from build123d import *
from build123d.topology import SkipClean

# Parameters (mm, degrees)
SKETCH_2_R             = 3
EXTRUDE_1_DEPTH        = 16.5
EXTRUDE_1_2_DEPTH      = 16.5
EXTRUDE_1_3_DEPTH      = 16.5
EXTRUDE_1_4_DEPTH      = 16.5
SKETCH_3_R             = 1.2
EXTRUDE_2_DEPTH        = 5
SKETCH_4_R             = 5
EXTRUDE_3_DEPTH        = 3
EXTRUDE_3_2_DEPTH      = 3
EXTRUDE_3_3_DEPTH      = 3
EXTRUDE_3_4_DEPTH      = 3
EXTRUDE_4_DEPTH        = 3
EXTRUDE_4_DEPTH_BACK   = 15
SKETCH_6_R             = 5
EXTRUDE_5_DEPTH        = 3
EXTRUDE_5_DEPTH_BACK   = 15
EXTRUDE_5_2_DEPTH      = 3
EXTRUDE_5_2_DEPTH_BACK = 15
EXTRUDE_6_DEPTH        = 3
SKETCH_9_R             = 1.9
EXTRUDE_7_DEPTH        = 4
SKETCH_10_R            = 1.9
EXTRUDE_8_DEPTH        = 4
CHAMFER_1_SIZE         = 1
SKETCH_11_R            = 5
EXTRUDE_9_DEPTH        = 5
SKETCH_12_R            = 2.1
CUT_EXTRUDE_1_DEPTH    = 5
SKETCH_13_R            = 2.1
CUT_EXTRUDE_2_DEPTH    = 4
CHAMFER_2_SIZE         = 1
CHAMFER_3_SIZE         = 0.5


with BuildPart() as part:
    # Sketch 2 → Extrude 1 (new body)
    with BuildSketch(Plane(origin=(0, 0, 0), x_dir=(1, 0, 0), z_dir=(0, 1, 0))):
        with Locations(Location((25, 35, 0), (0, 0, 270))):
            Circle(SKETCH_2_R)
    extrude(amount=EXTRUDE_1_DEPTH)



with BuildPart() as body_2:
    # Sketch 2 → Extrude 1 2 (new body)
    with BuildSketch(Plane(origin=(0, 0, 0), x_dir=(1, 0, 0), z_dir=(0, 1, 0))):
        with Locations(Location((31, -22, 0), (0, 0, 270))):
            Circle(SKETCH_2_R)
    extrude(amount=EXTRUDE_1_2_DEPTH)


with BuildPart() as body_3:
    # Sketch 2 → Extrude 1 3 (new body)
    with BuildSketch(Plane(origin=(0, 0, 0), x_dir=(1, 0, 0), z_dir=(0, 1, 0))):
        with Locations(Location((-31, -22, 0), (0, 0, 90))):
            Circle(SKETCH_2_R)
    extrude(amount=EXTRUDE_1_3_DEPTH)


with BuildPart() as body_4:
    # Sketch 2 → Extrude 1 4 (new body)
    with BuildSketch(Plane(origin=(0, 0, 0), x_dir=(1, 0, 0), z_dir=(0, 1, 0))):
        with Locations(Location((-25, 35, 0), (0, 0, 90))):
            Circle(SKETCH_2_R)
    extrude(amount=EXTRUDE_1_4_DEPTH)


with BuildPart() as part_1:
    add(part.part)

    add(body_2.part)  # Extrude 2 merges body 2

    add(body_3.part)  # Extrude 2 merges body 3

    add(body_4.part)  # Extrude 2 merges body 4
    # Sketch 3 → Extrude 2 (add)
    with BuildSketch(Plane(origin=(0, 16.5, 0), x_dir=(1, 0, 0), z_dir=(0, 1, 0))):
        with Locations(Location((-31, -22, 0), (0, 0, 270))):
            Circle(SKETCH_3_R)
        with Locations(Location((-25, 35, 0), (0, 0, 270))):
            Circle(SKETCH_3_R)
        with Locations(Location((25, 35, 0), (0, 0, 270))):
            Circle(SKETCH_3_R)
        with Locations(Location((31, -22, 0), (0, 0, 270))):
            Circle(SKETCH_3_R)
    extrude(amount=EXTRUDE_2_DEPTH)

    # Sketch 6 → Extrude 4 (add, two sides: drawn at the far end of the back side and taken through both)
    with BuildSketch(Plane(origin=(0, 0, 0), x_dir=(1, 0, 0), z_dir=(0, 1, 0)).offset(-EXTRUDE_4_DEPTH_BACK)):
        with Locations(Location((-28.159807037, -19, 0), (0, 0, 270))):
            Circle(SKETCH_6_R)
        with Locations(Location((28.159807037, -19, 0), (0, 0, 276.602489978))):
            Circle(SKETCH_6_R)
    extrude(amount=EXTRUDE_4_DEPTH + EXTRUDE_4_DEPTH_BACK)



with BuildPart() as body_2_2:
    # Sketch 4 → Extrude 3 (new body)
    with BuildSketch(Plane.XZ):
        with Locations(Location((-25, -15, 0), (0, 0, 270))):
            Circle(SKETCH_4_R)
    extrude(amount=-EXTRUDE_3_DEPTH)


with BuildPart() as body_3_2:
    # Sketch 4 → Extrude 3 2 (new body)
    with BuildSketch(Plane.XZ):
        with Locations(Location((-25, -75, 0), (0, 0, 270))):
            Circle(SKETCH_4_R)
    extrude(amount=-EXTRUDE_3_2_DEPTH)


with BuildPart() as body_4_2:
    # Sketch 4 → Extrude 3 3 (new body)
    with BuildSketch(Plane.XZ):
        with Locations(Location((25, -15, 0), (0, 0, 90))):
            Circle(SKETCH_4_R)
    extrude(amount=-EXTRUDE_3_3_DEPTH)


with BuildPart() as body_5:
    # Sketch 4 → Extrude 3 4 (new body)
    with BuildSketch(Plane.XZ):
        with Locations(Location((33, -75, 0), (0, 0, 270))):
            Circle(SKETCH_4_R)
    extrude(amount=-EXTRUDE_3_4_DEPTH)


with BuildPart() as body_6:
    # Sketch 7 → Extrude 5 (new, two sides: drawn at the far end of the back side and taken through both)
    with BuildSketch(Plane(origin=(0, 0, 0), x_dir=(1, 0, 0), z_dir=(0, 1, 0)).offset(-EXTRUDE_5_DEPTH_BACK)):
        with BuildLine():
            Line((32.175491387, -57.49808516), (25.273954776, -60.367671435))
            ThreePointArc((25.273954776, -60.367671435), (31.919625632, -66.61682114), (32.175491387, -57.49808516))
        make_face()
    extrude(amount=EXTRUDE_5_DEPTH + EXTRUDE_5_DEPTH_BACK)


with BuildPart() as body_7:
    # Sketch 7 → Extrude 5 2 (new, two sides: drawn at the far end of the back side and taken through both)
    with BuildSketch(Plane(origin=(0, 0, 0), x_dir=(1, 0, 0), z_dir=(0, 1, 0)).offset(-EXTRUDE_5_2_DEPTH_BACK)):
        with BuildLine():
            Line((-25.273954776, -60.367671435), (-32.175491387, -57.49808516))
            ThreePointArc((-32.175491387, -57.49808516), (-31.919625632, -66.61682114), (-25.273954776, -60.367671435))
        make_face()
    extrude(amount=EXTRUDE_5_2_DEPTH + EXTRUDE_5_2_DEPTH_BACK)


with BuildPart() as part_2:
    add(part_1.part)

    add(body_2_2.part)  # Extrude 6 merges body 2 2

    add(body_3_2.part)  # Extrude 6 merges body 3 2

    add(body_4_2.part)  # Extrude 6 merges body 4 2

    add(body_5.part)  # Extrude 6 merges body 5

    add(body_6.part)  # Extrude 6 merges body 6

    add(body_7.part)  # Extrude 6 merges body 7
    # Sketch 8 → Extrude 6 (add)
    with BuildSketch(Plane(origin=(0, 0, 0), x_dir=(1, 0, 0), z_dir=(0, 1, 0))):
        with BuildLine():
            Line((38.5, -33.396121926), (38.5, -56.841295093))
            Line((38.5, -56.841295093), (33.828278981, -58.783747516))
            ThreePointArc((33.828278981, -58.783747516), (34.61682114, -60.080374368), (34.98005436, -61.5538402))
            Line((34.98005436, -61.5538402), (41.5, -58.842915434))
            Line((41.5, -58.842915434), (41.5, -32.2880886))
            Line((41.5, -32.2880886), (32.400068827, -21.64956222))
            ThreePointArc((32.400068827, -21.64956222), (31.409890316, -22.799599805), (30.120308944, -23.599612187))
            Line((30.120308944, -23.599612187), (38.5, -33.396121926))
        make_face()
        with BuildLine():
            Line((-41.5, -32.2880886), (-41.5, -58.842915434))
            Line((-41.5, -58.842915434), (-34.98005436, -61.5538402))
            ThreePointArc((-34.98005436, -61.5538402), (-34.61682114, -60.080374368), (-33.828278981, -58.783747516))
            Line((-33.828278981, -58.783747516), (-38.5, -56.841295093))
            Line((-38.5, -56.841295093), (-38.5, -33.396121926))
            Line((-38.5, -33.396121926), (-30.120308944, -23.599612187))
            ThreePointArc((-30.120308944, -23.599612187), (-31.409890316, -22.799599805), (-32.400068827, -21.64956222))
            Line((-32.400068827, -21.64956222), (-41.5, -32.2880886))
        make_face()
        with BuildLine():
            ThreePointArc((26.224871012, -14.389574577), (27.697123337, -14.021453647), (29.211998824, -14.111964357))
            Line((29.211998824, -14.111964357), (26.934936025, 10.389574577))
            ThreePointArc((26.934936025, 10.389574577), (25.4626837, 10.021453647), (23.947808213, 10.111964357))
            Line((23.947808213, 10.111964357), (26.224871012, -14.389574577))
        make_face()
        with BuildLine():
            ThreePointArc((23.5, 19.769696007), (25, 20), (26.5, 19.769696007))
            Line((26.5, 19.769696007), (26.5, 32.401923789))
            ThreePointArc((26.5, 32.401923789), (25, 32), (23.5, 32.401923789))
            Line((23.5, 32.401923789), (23.5, 19.769696007))
        make_face()
        with BuildLine():
            Line((-20.230303993, 13.5), (20.230303993, 13.5))
            ThreePointArc((20.230303993, 13.5), (20, 15), (20.230303993, 16.5))
            Line((20.230303993, 16.5), (-20.230303993, 16.5))
            ThreePointArc((-20.230303993, 16.5), (-20, 15), (-20.230303993, 13.5))
        make_face()
        with BuildLine():
            Line((-26.224871012, -14.389574577), (-23.947808213, 10.111964357))
            ThreePointArc((-23.947808213, 10.111964357), (-25.4626837, 10.021453647), (-26.934936025, 10.389574577))
            Line((-26.934936025, 10.389574577), (-29.211998824, -14.111964357))
            ThreePointArc((-29.211998824, -14.111964357), (-27.697123337, -14.021453647), (-26.224871012, -14.389574577))
        make_face()
        with BuildLine():
            ThreePointArc((24.038653652, 37.84179753), (25.588348405, 37.941742027), (26.980395679, 37.253449124))
            Line((26.980395679, 37.253449124), (33.535456667, 70.028754064))
            ThreePointArc((33.535456667, 70.028754064), (32.019419324, 70.097096622), (30.59371464, 70.617102469))
            Line((30.59371464, 70.617102469), (24.038653652, 37.84179753))
        make_face()
        with BuildLine():
            ThreePointArc((-26.5, 19.769696007), (-25, 20), (-23.5, 19.769696007))
            Line((-23.5, 19.769696007), (-23.5, 32.401923789))
            ThreePointArc((-23.5, 32.401923789), (-25, 32), (-26.5, 32.401923789))
            Line((-26.5, 32.401923789), (-26.5, 19.769696007))
        make_face()
        with BuildLine():
            Line((-20.230303993, 73.5), (28.230303993, 73.5))
            ThreePointArc((28.230303993, 73.5), (28, 75), (28.230303993, 76.5))
            Line((28.230303993, 76.5), (-20.230303993, 76.5))
            ThreePointArc((-20.230303993, 76.5), (-20, 75), (-20.230303993, 73.5))
        make_face()
        with BuildLine():
            Line((-26.5, 70.230303993), (-26.5, 37.598076211))
            ThreePointArc((-26.5, 37.598076211), (-25, 38), (-23.5, 37.598076211))
            Line((-23.5, 37.598076211), (-23.5, 70.230303993))
            ThreePointArc((-23.5, 70.230303993), (-25, 70), (-26.5, 70.230303993))
        make_face()
    extrude(amount=EXTRUDE_6_DEPTH)

    # Sketch 9 → Extrude 7 (add)
    with BuildSketch(Plane.XZ.offset(15)):
        with Locations(Location((28.159807037, 19, 0), (0, 0, 270))):
            Circle(SKETCH_9_R)
        with Locations(Location((30, 62, 0), (0, 0, 270))):
            Circle(SKETCH_9_R)
        with Locations(Location((-28.159807037, 19, 0), (0, 0, 90))):
            Circle(SKETCH_9_R)
        with Locations(Location((-30, 62, 0), (0, 0, 90))):
            Circle(SKETCH_9_R)
    extrude(amount=EXTRUDE_7_DEPTH)

    # Sketch 10 → Extrude 8 (add)
    with BuildSketch(Plane.XZ):
        with Locations(Location((25, -15, 0), (0, 0, 90))):
            Circle(SKETCH_10_R)
        with Locations(Location((33, -75, 0), (0, 0, 90))):
            Circle(SKETCH_10_R)
        with Locations(Location((-25, -75, 0), (0, 0, 90))):
            Circle(SKETCH_10_R)
        with Locations(Location((-25, -15, 0), (0, 0, 90))):
            Circle(SKETCH_10_R)
    extrude(amount=EXTRUDE_8_DEPTH)

    # Chamfer 1
    chamfer_1_edges = [part_2.edges().sort_by_distance(p)[0] for p in [
        (28.159807037, -19, 20.9),
        (30, -19, 63.9),
        (-28.159807037, -19, 17.1),
        (-30, -19, 60.1),
        (25, -4, -16.9),
        (33, -4, -76.9),
        (-25, -4, -76.9),
        (-25, -4, -16.9),
    ]]
    chamfer(chamfer_1_edges, length=CHAMFER_1_SIZE)

    # Sketch 11 → Extrude 9 (add)
    with SkipClean():  # the faces are left unmerged after this step: merging them gives an invalid solid
        with BuildSketch(Plane(origin=(0, 3, 0), x_dir=(1, 0, 0), z_dir=(0, 1, 0))):
            with Locations(Location((33, 75, 0), (0, 0, 162.542396876))):
                Circle(SKETCH_11_R)
            with Locations(Location((-25, 75, 0), (0, 0, 17.457603124))):
                Circle(SKETCH_11_R)
        extrude(amount=EXTRUDE_9_DEPTH)
    add(part_2.part.scale(1), mode=Mode.REPLACE)  # the faces are merged on a copy

    # Sketch 12 → Cut-Extrude 1 (cut)
    with BuildSketch(Plane(origin=(0, 3, 0), x_dir=(1, 0, 0), z_dir=(0, 1, 0))):
        with Locations(Location((30, -62, 0), (0, 0, 270))):
            Circle(SKETCH_12_R)
        with Locations(Location((-30, -62, 0), (0, 0, 90))):
            Circle(SKETCH_12_R)
    extrude(amount=-CUT_EXTRUDE_1_DEPTH, mode=Mode.SUBTRACT)

    # Sketch 13 → Cut-Extrude 2 (cut)
    with BuildSketch(Plane(origin=(0, 8, 0), x_dir=(1, 0, 0), z_dir=(0, 1, 0))):
        with Locations(Location((33, 75, 0), (0, 0, 270))):
            Circle(SKETCH_13_R)
        with Locations(Location((-25, 75, 0), (0, 0, 270))):
            Circle(SKETCH_13_R)
    extrude(amount=-CUT_EXTRUDE_2_DEPTH, mode=Mode.SUBTRACT)

    # Chamfer 2
    chamfer_2_edges = [part_2.edges().sort_by_distance(p)[0] for p in [
        (30, 3, 59.9),
        (-30, 3, 64.1),
        (33, 8, -77.1),
        (-25, 8, -77.1),
    ]]
    chamfer(chamfer_2_edges, length=CHAMFER_2_SIZE)

    # Chamfer 3
    chamfer_3_edges = [part_2.edges().sort_by_distance(p)[0] for p in [
        (31, 16.5, 20.8),
        (31, 21.5, 20.8),
        (-31, 16.5, 20.8),
        (-31, 21.5, 20.8),
        (25, 16.5, -36.2),
        (25, 21.5, -36.2),
        (-25, 16.5, -36.2),
        (-25, 21.5, -36.2),
    ]]
    chamfer(chamfer_3_edges, length=CHAMFER_3_SIZE)


solid = part_2.part
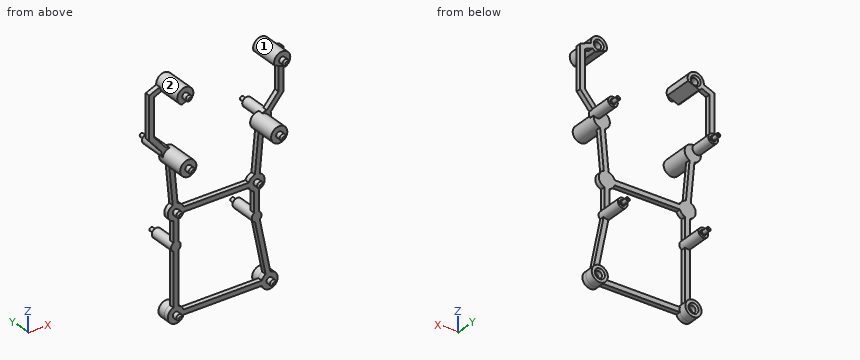
Model file for the job. Use its own axes, mm. Face numbers are marked on the shaded views. Give positions to 0.01 mm unless a question says otherwise; leave off trailing zeros. Loops run counter-clockwise (first coordinate to the right, second up) from the corner with the lowest first, then second, coordinate; pieces in that order, holes last. Notation, with made-up numbers: (65.25, -5.5) - (83.25, -5.5) arc R23 ccw to (83.25, 2.5) - close; hole circle Ø3 at (-29.75, 70.5). An arc over 180 degrees is marked (long way). Use one line per item in the form item = value.
(1) Drop flat-ended pins along their axis: P1, Ø5.5, axis at x = 30, z = 62, coming from the +Y side; P2, Ø2, axis at x = -24, y = -5.5, coming from the -Z side (3 decimals); P3, Ø3.5, axis at y = 1, z = -23.5, coming from the -X side. Give the stop position or say it passes through.
Determined:
P1 = 2.65
P2 = 15.125
P3 = -26.5
(2) Cut at A-A (x = -11). Give the cut face in (y, z), then the cut area to 3 significant figures.
Determined:
outline = (0, -76.5) - (3, -76.5) - (3, -73.5) - (0, -73.5) - close; (0, -16.5) - (3, -16.5) - (3, -13.5) - (0, -13.5) - close
area = 18.0 mm^2
(3) Drill centre lines: L1, parallel to X at y = -1, z = 62; L2, parallel to X at y = 5.35, z = -75; L3, parallel to Y at x = -9.5, z = -15. Where is each one in solid material? Low to high.
Determined:
L1 = -35 to -32.1, -27.9 to -25, 25 to 27.9, 32.1 to 35
L2 = -30 to -27.1, -22.9 to -20, 28 to 30.9, 35.1 to 38
L3 = 0 to 3
(4) Pull direction X, two halves, no side cores. Call the marked faces 1 and 2: pulls with the +X half, pulls with the -X half, needs draft (parallel to the pull), parting line crosses it, or undercut.
Determined:
face_1 = undercut
face_2 = undercut
(5) Cut at C-C (y = -9). Give the cut face in (x, z), then the cut area to 3 significant figures.
Determined:
outline = circle Ø10 at (-28.16, 19); (-32.18, 57.5) - (-25.27, 60.37) arc R5 ccw (long way) to start; circle Ø10 at (28.16, 19); (25.27, 60.37) - (32.18, 57.5) arc R5 ccw (long way) to start
area = 297 mm^2
(6) Cut at B-B (z = 55). Give the cut face in (x, y), then the cut area to 3 significant figures.
Determined:
outline = (-41.5, 0) - (-38.5, 0) - (-38.5, 3) - (-41.5, 3) - close; (38.5, 0) - (41.5, 0) - (41.5, 3) - (38.5, 3) - close
area = 18.0 mm^2
